Can you work these out from the model? Positions are in its coordinate system, mm. A direction names the side the tool comes from. Coordinates: 2 decimals unless noted, no trailing zeros. Write each loop counter-clockwise with the first axis right and the second up, starting at its lowest first coordinate (ties: lowest second). Pieces come first, ordered by that corner, then holes. Notation, with made-up numbers: (50, 35.25) -> (77, 35.25) arc R20 ccw to (77, 46.25) -> close; hole circle Ø2 at (41, 3). An arc over 180 degrees is marked (long way). Use one line per item in the form item = value.
```python
from build123d import *

# Parameters (mm, degrees)
PAD_DEPTH       = 10
POCKET_DEPTH    = 3.1
SKETCH002_R     = 1.6
POCKET001_DEPTH = 4.201
CHAMFER_SIZE    = 0.4
CHAMFER001_SIZE = 0.2
FILLET_R        = 0.6


with BuildPart() as part:
    # Sketch → Pad (new body)
    with BuildSketch(Plane.XZ):
        Polygon((-5.3, 0), (5.3, 0), (5.3, 1.4), (2.5, 4.2), (-2.5, 4.2), (-5.3, 1.4), align=None)
    extrude(amount=PAD_DEPTH)

    # Sketch001 → Pocket (cut)
    with BuildSketch(Plane(origin=(0, 0, 4.2), x_dir=(-1, 0, 0), z_dir=(0, 0, 1))):
        Polygon((1.6, 2.228719), (3.2, 5), (1.6, 7.771281), (-1.6, 7.771281), (-3.2, 5), (-1.6, 2.228719), align=None)
    extrude(amount=-POCKET_DEPTH, mode=Mode.SUBTRACT)

    # Sketch002 → Pocket001 (cut, through all)
    with BuildSketch(Plane(origin=(0, 0, 0), x_dir=(1, 0, 0), z_dir=(0, 0, -1))):
        with Locations((0, 5)):
            Circle(SKETCH002_R)
    extrude(amount=-POCKET001_DEPTH, mode=Mode.SUBTRACT)

    # Chamfer
    chamfer_edges = [part.edges().sort_by_distance(p)[0] for p in [
        (-1.6, -5, 0),
    ]]
    chamfer(chamfer_edges, length=CHAMFER_SIZE)

    # Chamfer001
    chamfer001_edges = [part.edges().sort_by_distance(p)[0] for p in [
        (-5.3, -5, 0),
        (5.3, -5, 0),
    ]]
    chamfer(chamfer001_edges, length=CHAMFER001_SIZE)

    # Fillet
    fillet_edges = [part.edges().sort_by_distance(p)[0] for p in [
        (-5.3, 0, 0.8),
        (5.3, 0, 0.8),
        (-3.9, 0, 2.8),
        (3.9, 0, 2.8),
        (0, 0, 4.2),
        (-5.3, -10, 0.8),
        (5.3, -10, 0.8),
        (-3.9, -10, 2.8),
        (3.9, -10, 2.8),
        (0, -10, 4.2),
    ]]
    fillet(fillet_edges, radius=FILLET_R)


solid = part.part
```
Q1. Suppose I cut it at C-C (y = -8). Write out the boundary of the cut face in (x, z), then the cut area to 3 significant figures.
Return value:
outline = (-5.3, 0.2) -> (-5.1, 0) -> (5.1, 0) -> (5.3, 0.2) -> (5.3, 1.4) -> (2.5, 4.2) -> (-2.5, 4.2) -> (-5.3, 1.4) -> close
area = 36.6 mm2
Q2. For faces 1 (the flat face through (0, -7.771, 3)), 2 (the flat face through (0, 0, 1)), which set-ups out of +Z, -Z, +X, -X, +Y, -Y let a thin tool reach every point of the face, with its end or its side?
Return value:
face_1 = +Z
face_2 = +Z, -Z, +X, -X, +Y
Q3. Suppose I cut it at B-B (z = 0.7). Write out the boundary of the cut face in (x, y), then the cut area to 3 significant figures.
Return value:
outline = (-5.3, -9.4) arc R0.6 ccw to (-4.7, -10) -> (4.7, -10) arc R0.6 ccw to (5.3, -9.4) -> (5.3, -0.6) arc R0.6 ccw to (4.7, 0) -> (-4.7, 0) arc R0.6 ccw to (-5.3, -0.6) -> close; hole circle Ø3.2 at (0, -5)
area = 97.6 mm2
Q4. Suppose I cut it at A-A (x = 0). Write out the boundary of the cut face in (y, z), then the cut area to 3 significant figures.
Return value:
outline = (-10, 0) -> (-7, 0) -> (-6.6, 0.4) -> (-6.6, 1.1) -> (-7.77, 1.1) -> (-7.77, 4.2) -> (-9.4, 4.2) arc R0.6 ccw to (-10, 3.6) -> close; (-3.4, 0.4) -> (-3, 0) -> (0, 0) -> (0, 3.6) arc R0.6 ccw to (-0.6, 4.2) -> (-2.23, 4.2) -> (-2.23, 1.1) -> (-3.4, 1.1) -> close
area = 21.0 mm2
Q5. Thinking about a two-plate mould opening in X: for faces 3 (the flat face through (0, -2.229, 3)), 4 (the flat face through (-0.1, -2.7, 0)), 5 (the cylindrical face through (-3.79, -9.83, 2.65)), which applies, released by +X, released by -X, zero draft, split by the parting line, or undercut?
Return value:
face_3 = undercut
face_4 = zero draft
face_5 = released by -X
Q6. If I drill on line 1 (Y direction, x = -0.25, z = 3.4); line 2 (Y direction, x = 0, z = 0.75); line 3 (X direction, y = -5, z = 0.95), over which ranges is the centre line in solid material (lowest first)? Write a range as from..to.
Return value:
line_1 = -10..-7.77, -2.23..0
line_2 = -10..-6.6, -3.4..0
line_3 = -5.3..-1.6, 1.6..5.3
Q7. Will these pins go through, and if not, where does the flat tip stop? pin 1 (1.5 mm diameter, centred on y = -1, z = 3, fed in from +X); pin 2 (1 mm diameter, centred on x = -1, y = -6, fed in from +Z).
Return value:
pin_1 = 4.45
pin_2 = 1.1
